Autodesk Inventor part; units mm, degrees
ref_plane "YZ Plane" through (0, 0, 0) normal (1, 0, 0) x (0, 1, 0)
ref_plane "XZ Plane" through (0, 0, 0) normal (0, 1, 0) x (-1, 0, 0)
ref_plane "XY Plane" through (0, 0, 0) normal (0, 0, 1) x (1, 0, 0)
sketch "Sketch1" plane through (0, 0, 0) normal (0, 1, 0) x (-1, 0, 0)
  circle A0 centre (0, 0) radius 50.8
  dimension "d0" = 101.6
extrude "Extrusion1" add sketch "Sketch1" along normal blind 38.1
sketch "Sketch2" plane through (0, 38.1, 0) normal (0, 1, 0) x (1, 0, 0)
  point P0 (0, 0)
  point P1 (-31.75, 0)
  point P2 (-9.8113, -30.196)
  point P3 (25.6863, -18.6622)
  point P4 (25.6863, 18.6622)
  point P5 (-9.8113, 30.196)
  dimension "d3" = 31.75
  dimension "d4" = 0
  dimension "d7" = 360
hole "Hole1" at (-31.75, 38.1, 0) direction (0, -1, 0) diameter 6.35 end through all
hole "Hole2" at (-9.8113, 38.1, 30.196) direction (0, -1, 0) diameter 9.525 end through all counterbore diameter 19.05 counterbore depth 6.35
hole "Hole3" at (25.6863, 38.1, 18.6622) direction (0, -1, 0) diameter 9.525 end through all countersink diameter 19.05 countersink angle 82
hole "Hole4" at (-9.8113, 38.1, -30.196) direction (0, -1, 0) diameter 4.9784 end through all countersink diameter 19.05 countersink angle 82
hole "Hole5" at (25.6863, 38.1, -18.6622) direction (0, -1, 0) diameter 13.4874 end through all
properties part number "Hole Practice"
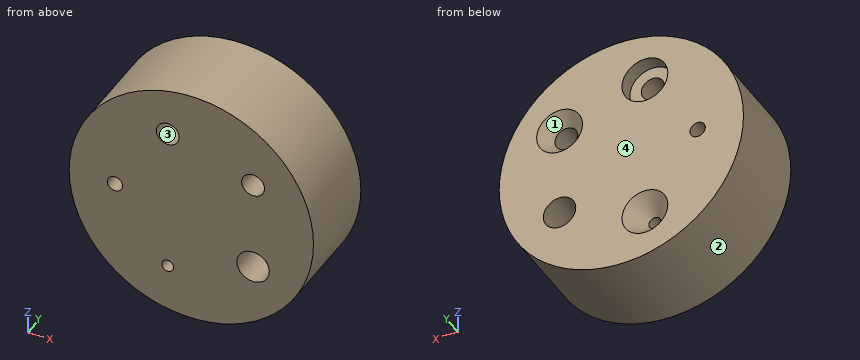
Design review of the part built by this model. Coordinates are the model's own, in mm. Face numbers are marked on the shaded views. Give positions to 0.01 mm unless a question says otherwise; leave off trailing zeros. Order: outer loops, then holes, each group sorted by start corner. A loop starts at its lowest first (then second) coordinate and runs counter-clockwise, first axis right, second up. Notation, with made-up numbers: (56.25, -26.5) -> (89.25, -26.5) arc R24 cw to (89.25, -3.5) -> close; hole circle Ø11 at (41.5, 32). An arc over 180 degrees is marked (long way). Write each question's results on one line, items separated by ' | '. Start each with the question number.
Q1. Wall thickness on L1, parallel to Z at x = -8.5, y = 4; L2, parallel to Z at x = -13.5, y = 23; L3, parallel to Z at x = 21.5, y = 8.5: over which ranges is each line inside the solid? List them lowest first. Write a range as from..to.
Q2. Mouldability with a two-part tool opening along X and no side actions: class the marked faces 1, 2, 3 and 4 as +X half, -X half, draft (parallel to the pull), parting line (faces both ways), or undercut.
Q3. Add section C-C on y = 9. State how many separate pieces and enclosed holes the cut face has, and give its area (3 significant figures).
Q4. Add section D-D on x = 13. Give the boundary of the cut face in (y, z), and give its area (3 significant figures).
Q5. Add section A-A on z = 0. Give the boundary of the cut face in (x, y) (3 decimals), and give its area (3 significant figures).
Q6. For pin 1 (11 mm diameter, centred on x = 25.69, z = 18.66, fed in from +Y); pin 2 (3 mm diameter, centred on x = -9.81, z = -30.2, fed in from -Y); pin 3 (12 mm diameter, centred on y = 24.5, z = 27, fed in from -X); pin 4 (10 mm diameter, centred on x = 15, y = 19, fed in from +Z), all flat-tipped, find the tip position at first contact; note any pin that passes through.
Q7. Add section B-B on x = -31.75. Give the boundary of the cut face in (y, z) (3 decimals), and give its area (3 significant figures).
Found:
1) L1: z = -50.08..-32.31, -28.08..25.62, 34.77..50.08 | L2: z = -48.97..27.18, 33.21..48.97 | L3: z = -46.03..-23.95, -13.38..16.39, 20.93..46.03
2) face 1: undercut | face 2: parting line | face 3: undercut | face 4: draft
3) separate pieces: 1 | enclosed holes: 5 | area: 7,770 mm2
4) outline: (0, -49.11) -> (38.1, -49.11) -> (38.1, 49.11) -> (0, 49.11) -> close | area: 3,740 mm2
5) outline: (-50.8, 0) -> (-34.925, 0) -> (-34.925, 38.1) -> (-50.8, 38.1) -> close; (-28.575, 0) -> (50.8, 0) -> (50.8, 38.1) -> (-28.575, 38.1) -> close | area: 3,630 mm2
6) pin 1: stops at y = 33.47 | pin 2: passes through | pin 3: stops at x = -46.26 | pin 4: stops at z = 49.81
7) outline: (0, -39.656) -> (38.1, -39.656) -> (38.1, -3.175) -> (0, -3.175) -> close; (0, 3.175) -> (38.1, 3.175) -> (38.1, 39.656) -> (0, 39.656) -> close | area: 2,780 mm2
